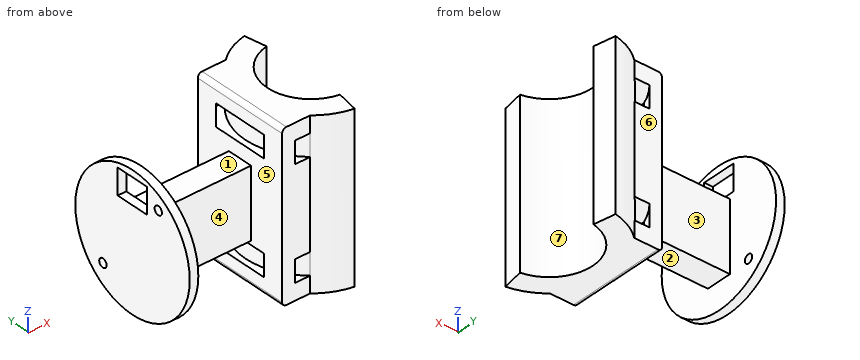
```python
from build123d import *

# Parameters (mm, degrees)
BOSS_EXTRUDE1_DEPTH = 19.05
SKETCH6_W           = 16.071399664
SKETCH6_H           = 6
BOSS_EXTRUDE3_DEPTH = 23
SKETCH3_W           = 2.54
SKETCH3_H           = 5.08
SKETCH4_R           = 15.5
SKETCH4_R_2         = 1
SKETCH4_W           = 8
SKETCH4_H           = 6
BOSS_EXTRUDE2_DEPTH = 2
FILLET1_R           = 1


with BuildPart() as part:
    # Sketch1 → Boss-Extrude1 (new body, symmetric)
    with BuildSketch(Plane.XY):
        with BuildLine():
            Line((8.346153406, -9.946558305), (7.464020663, -14.949381691))
            ThreePointArc((7.464020663, -14.949381691), (3.546652059, -13.692553844), (0.110630651, -11.43))
            Line((0.110630651, -11.43), (-6.389369349, -11.43))
            Line((-6.389369349, -11.43), (-6.389369349, 11.43))
            Line((-6.389369349, 11.43), (0.110630651, 11.43))
            ThreePointArc((0.110630651, 11.43), (3.546652059, 13.692553844), (7.464020663, 14.949381691))
            Line((7.464020663, 14.949381691), (8.346153406, 9.946558305))
            ThreePointArc((8.346153406, 9.946558305), (0, 0), (8.346153406, -9.946558305))
        make_face()
    extrude(amount=BOSS_EXTRUDE1_DEPTH, both=True)

    # Sketch6 → Boss-Extrude3 (add)
    with BuildSketch(Plane.ZY.offset(6.389369349)):
        with Locations((-1.213689559, 0)):
            Rectangle(SKETCH6_W, SKETCH6_H)
    extrude(amount=BOSS_EXTRUDE3_DEPTH)

    # Sketch3 → Cut-Revolve1 (revolve, cut)
    with BuildSketch(Plane(origin=(0, 0, 0), x_dir=(1, 0, 0), z_dir=(0, 1, 0))):
        with Locations((-6.35, 12.7)):
            Rectangle(SKETCH3_W, SKETCH3_H)
        with Locations((-6.35, -12.7)):
            Rectangle(SKETCH3_W, SKETCH3_H)
    revolve(axis=Axis((10.1, 0, 19.05), (0, 0, -1)), mode=Mode.SUBTRACT)

    # Sketch4 → Boss-Extrude2 (add)
    with BuildSketch(Plane(origin=(-29.389369349, 0, 0), x_dir=(0, -1, 0), z_dir=(-1, 0, 0))):
        Circle(SKETCH4_R)
        with Locations((6.97426488, 10.435972737)):
            Circle(SKETCH4_R_2, mode=Mode.SUBTRACT)
        with Locations((-8.02573512, -8.580948715)):
            Circle(SKETCH4_R_2, mode=Mode.SUBTRACT)
        with Locations((-0.025715642, 10.93618237)):
            Rectangle(SKETCH4_W, SKETCH4_H, mode=Mode.SUBTRACT)
    extrude(amount=BOSS_EXTRUDE2_DEPTH)

    # Fillet1
    fillet1_edges = [part.edges().sort_by_distance(p)[0] for p in [
        (-6.389369349, 0, 19.05),
        (-6.389369349, 0, -19.05),
    ]]
    fillet(fillet1_edges, radius=FILLET1_R)


solid = part.part
```
Could you check a few things on this model? Use its own coordinates, in mm. Face numbers are marked on the shaded views. A direction names the side the tool comes from. Give positions to 0.01 mm unless a question says otherwise; leave off trailing zeros. Loops run counter-clockwise (first coordinate to the right, second up) from the corner with the lowest first, then second, coordinate; pieces in that order, holes last. Notation, with made-up numbers: (61.25, -39.75) - (89.25, -39.75) arc R13 ccw to (89.25, -19.75) - close; hole circle Ø8 at (47, -29.5). An arc over 180 degrees is marked (long way). Answer in a Markdown table with one row per item. Add a question column.
Q1. If we section it at A-A (y = 0): List the corners of the cut face in (x, z) for me.
Q2. If we section it at B-B (z = 0): List the corners of the cut face in (x, y) for me.
Q3. For pin 1 (4 mm diameter, centred on y = -0.5, z = 15, fed in from +X); pin 2 (3 mm diameter, centred on x = -21.5, y = 1, fed in from -Z); pin 3 (7 mm diameter, centred on x = -4, z = 3, fed in from -Y); pin 4 (6 mm diameter, centred on x = -25.5, y = 11.5, fed in from -Z), each with a flat end and sliding along its axis, tell me the tip position at first contact or that it passes through.
Q4. Which directions (+Z, -Z, +X, -X, +Y, -Y) give clear straight access to the entire face, cutting with the end or side of a thin tool? Please do the marked faces 1, 2, 3 and 4.
Q5. If we section it at D-D (y = 13.5): List the corners of the cut face in (x, z) for me.
Q6. We'd pull the mould along Y, two halves only. Please class the marked faces 5, 6 and 7: +Y half, -Y half, draft (parallel to the pull), parting line (faces both ways), or undercut.
Q7. Please list where these lines run through material, in increasing order: L1, parallel to Z at x = -4, y = 8; L2, parallel to X at y = 3.5, z = -12; L3, parallel to Y at x = 4, z = -10. Write a range as from..to.
Q8. If we section it at C-C (x = -16.5): List the corners of the cut face in (y, z) for me, plus the area to 3 significant figures.
The answers:
| question | item | result |
|---|---|---|
| 1 | outline | (-31.39, -15.5) - (-29.39, -15.5) - (-29.39, -9.25) - (-6.39, -9.25) - (-6.39, -10.16) - (-5.08, -10.16) - (-5.08, -15.24) - (-6.39, -15.24) - (-6.39, -18.05) arc R1 ccw to (-5.39, -19.05) - (0, -19.05) - (0, 19.05) - (-5.39, 19.05) arc R1 ccw to (-6.39, 18.05) - (-6.39, 15.24) - (-5.08, 15.24) - (-5.08, 10.16) - (-6.39, 10.16) - (-6.39, 6.82) - (-29.39, 6.82) - (-29.39, 7.94) - (-31.39, 7.94) - close; (-31.39, 13.94) - (-29.39, 13.94) - (-29.39, 15.5) - (-31.39, 15.5) - close |
| 2 | outline | (-31.39, -15.5) - (-29.39, -15.5) - (-29.39, -3) - (-6.39, -3) - (-6.39, -11.43) - (0.11, -11.43) arc R15.18 ccw to (7.46, -14.95) - (8.35, -9.95) arc R10.1 cw to (8.35, 9.95) - (7.46, 14.95) arc R15.18 ccw to (0.11, 11.43) - (-6.39, 11.43) - (-6.39, 3) - (-29.39, 3) - (-29.39, 15.5) - (-31.39, 15.5) - close |
| 3 | pin 1 | stops at x = 0.31 |
| 3 | pin 2 | stops at z = -9.25 |
| 3 | pin 3 | stops at y = -11.43 |
| 3 | pin 4 | passes through |
| 4 | face 1 | +Z, +Y, -Y |
| 4 | face 2 | -Z, +Y, -Y |
| 4 | face 3 | +Z, -Z, +Y |
| 4 | face 4 | +Z, -Z, -Y |
| 5 | outline | (-31.39, -7.62) - (-29.39, -7.62) - (-29.39, 7.62) - (-31.39, 7.62) - close; (3.16, -19.05) - (7.72, -19.05) - (7.72, 19.05) - (3.16, 19.05) - close |
| 6 | face 5 | draft |
| 6 | face 6 | +Y half |
| 6 | face 7 | undercut |
| 7 | L1 | z = -19.05..-15.24, -10.16..10.16, 15.24..19.05 |
| 7 | L2 | x = -31.39..-29.39, -4.67..0.63 |
| 7 | L3 | y = -13.9..-8.05, 8.05..13.9 |
| 8 | outline | (-3, -9.25) - (3, -9.25) - (3, 6.82) - (-3, 6.82) - close |
| 8 | area | 96.4 mm^2 |
